Autodesk Inventor part; units mm, degrees
ref_plane "YZ Plane" through (0, 0, 0) normal (1, 0, 0) x (0, 1, 0)
ref_plane "XZ Plane" through (0, 0, 0) normal (0, 1, 0) x (-1, 0, 0)
ref_plane "XY Plane" through (0, 0, 0) normal (0, 0, 1) x (1, 0, 0)
sketch "Sketch1" plane through (0, 0, 0) normal (0, 1, 0) x (-1, 0, 0)
  circle A0 centre (0, 0) radius 1
  dimension "d0" = 2
extrude "Extrusion1" add sketch "Sketch1" along normal blind 6
sketch "Sketch2" plane through (0, 6, 0) normal (0, 1, 0) x (1, 0, 0)
  circle A0 centre (0, 0) radius 2
  dimension "d3" = 4
extrude "Extrusion2" add sketch "Sketch2" along normal blind 2
sketch "Sketch3" plane through (0, 8, 0) normal (0, 1, 0) x (1, 0, 0)
  circle A0 centre (0, 0) radius 1 construction
  circle A1 centre (0, 0) radius 1 construction
  circle A2 centre (0, 0) radius 1
  line L0 (-0.9996, -0.0278) -> (-0.5239, 0.8518)
  line L1 (-0.5239, 0.8518) -> (0.4758, 0.8796)
  line L2 (0.4758, 0.8796) -> (0.9996, 0.0278)
  line L3 (0.9996, 0.0278) -> (0.5239, -0.8518)
  line L4 (0.5239, -0.8518) -> (-0.4758, -0.8796)
  line L5 (-0.4758, -0.8796) -> (-0.9996, -0.0278)
  dimension "d6" = 2
extrude "Extrusion3" cut sketch "Sketch3" against normal blind 1 contours L3 L4 L5 L0 L1 L2
fillet "Fillet1" radius 1 1 edges at (-2, 8, 0)
thread "Thread1"
properties part number "2x6mmScrew"
Design review of the part built by this model. Coordinates are the model's own, in mm. A direction names the side the tool comes from. Coordinates: 2 decimals unless noted, no trailing zeros. Order: outer loops, then holes, each group sorted by start corner. A loop starts at its lowest first (then second) coordinate and runs counter-clockwise, first axis right, second up.
1) Clearance check with flat-ended pins moving along their axes: pin 1 (1.5 mm diameter, centred on x = 1, y = 1.5, fed in from +Z); pin 2 (2 mm diameter, centred on y = 3, z = -1.5, fed in from -X). State where each tip first meets the part, or that it passes through.
2) Take a section at B-B, the plane y = 6.25. Give the boundary of the cut face in (x, z), and give its area (3 significant figures).
3) Take a section at A-A, the plane x = 0. Give the boundary of the cut face in (y, z), and give its area (3 significant figures).
4) Mouldability with a two-part tool opening along X and no side actions: class faces 1 (the cylindrical face through (-0.434, 6.493, -1.952)), 2 (the flat face through (0, 0, 0)), 3 (the flat face through (-0.765, 7.507, -0.406)), 4 (the flat face through (0.765, 7.507, 0.406)) as +X half, -X half, draft (parallel to the pull), parting line (faces both ways), or undercut.
5) Wall thickness on line 1 along Y through (x, z) = (0.4, -0.65); line 2 along Z through (x, y) = (0.1, 7.75); line 3 along X through (y, z) = (7.75, -0.65): over which ranges is each line inside the solid? List them lowest first.
6) Take a section at C-C, the plane y = 4.75. Give the boundary of the cut face in (x, z).
7) For faces 5 (the flat face through (0.734, 7.507, -0.46)), 6 (the flat face through (1, 6, 1)), list the 3-axis set-ups (+Z, -Z, +X, -X, +Y, -Y) from which the entire face can be reached by the end or side of a thin tool; tool diameter is ignored.
Returned:
1. pin 1: stops at z = 0.97
1. pin 2: stops at x = -0.87
2. outline: circle Ø4 at (0, 0)
2. area: 12.6 mm2
3. outline: (0, -1) - (6, -1) - (6, -2) - (7, -2) arc R1 ccw to (8, -1) - (8, -0.87) - (7, -0.87) - (7, 0.87) - (8, 0.87) - (8, 1) arc R1 ccw to (7, 2) - (6, 2) - (6, 1) - (0, 1) - close
3. area: 17.8 mm2
4. face 1: parting line
4. face 2: draft
4. face 3: undercut
4. face 4: undercut
5. line 1: y = 0 to 7
5. line 2: z = -1.66 to -0.87, 0.86 to 1.66
5. line 3: x = -1.53 to -0.63, 0.62 to 1.53
6. outline: circle Ø2 at (0, 0)
7. face 5: +Y
7. face 6: -Y
